Build history of the part. All positions in model axes, mm. A direction names the side the tool comes from. Round coordinates to 2 decimals unless told otherwise and drop trailing zeros. Write each loop counter-clockwise with the first axis right and the second up, starting at its lowest first coordinate (ties: lowest second). Pieces come first, ordered by that corner, then holes. Notation, with made-up numbers: (-3.5, -9) -> (19.5, -9) arc R19 cw to (19.5, 19) -> close; hole circle Ø11 at (-21, -36). An arc over 180 degrees is marked (long way). Answer in a Markdown table with one row per item.
```python
from build123d import *

# Parameters (mm, degrees)
F1_DEPTH = 26
F2_DEPTH = 1.6


with BuildPart() as f1:
    # F0 (on Top) → F1 (new body)
    with BuildSketch(Plane.XY):
        with BuildLine():
            ThreePointArc((54.416171, 57.216655), (0, 61.6), (-54.416171, 57.216655))
            ThreePointArc((-54.416171, 57.216655), (-55.980157, 56.335105), (-56.6, 54.650179))
            Line((-56.6, 54.650179), (-56.6, -54.5))
            ThreePointArc((-56.6, -54.5), (-55.838478, -56.338478), (-54, -57.1))
            Line((-54, -57.1), (54, -57.1))
            ThreePointArc((54, -57.1), (55.838478, -56.338478), (56.6, -54.5))
            Line((56.6, -54.5), (56.6, 54.650179))
            ThreePointArc((56.6, 54.650179), (55.980157, 56.335105), (54.416171, 57.216655))
        make_face()
        with BuildLine():
            Line((54, -55.5), (-54, -55.5))
            ThreePointArc((-54, -55.5), (-54.707107, -55.207107), (-55, -54.5))
            Line((-55, -54.5), (-55, 54.650179))
            ThreePointArc((-55, 54.650179), (-54.761599, 55.298228), (-54.160066, 55.637285))
            ThreePointArc((-54.160066, 55.637285), (0, 60), (54.160066, 55.637285))
            ThreePointArc((54.160066, 55.637285), (54.761599, 55.298228), (55, 54.650179))
            Line((55, 54.650179), (55, -54.5))
            ThreePointArc((55, -54.5), (54.707107, -55.207107), (54, -55.5))
        make_face(mode=Mode.SUBTRACT)
    extrude(amount=F1_DEPTH)

    # F0 (on Top) → F2 (join)
    with BuildSketch(Plane.XY):
        with BuildLine():
            ThreePointArc((-55, -54.5), (-54.707107, -55.207107), (-54, -55.5))
            Line((-54, -55.5), (54, -55.5))
            ThreePointArc((54, -55.5), (54.707107, -55.207107), (55, -54.5))
            Line((55, -54.5), (55, 54.650179))
            ThreePointArc((55, 54.650179), (54.761599, 55.298228), (54.160066, 55.637285))
            ThreePointArc((54.160066, 55.637285), (0, 60), (-54.160066, 55.637285))
            ThreePointArc((-54.160066, 55.637285), (-54.761599, 55.298228), (-55, 54.650179))
            Line((-55, 54.650179), (-55, -54.5))
        make_face()
    extrude(amount=F2_DEPTH)


solid = f1.part
```
Q1. Saw through at B-B on y = 49. Write the cut outline in (x, z).
A:
| item | result |
|---|---|
| outline | (-56.6, 0) -> (56.6, 0) -> (56.6, 26) -> (55, 26) -> (55, 1.6) -> (-55, 1.6) -> (-55, 26) -> (-56.6, 26) -> close |
Q2. Two-plate mould, pull along Y, no slides. Class faces 3 (the cylindrical face through (-55.859, -56.318, 12.818)), 4 (the flat face through (56.6, -1, 13)), 5 (the flat face through (1, -55.5, 14)): released by +Y, released by -Y, zero draft, split by the parting line, or undercut.
A:
| item | result |
|---|---|
| face 3 | released by -Y |
| face 4 | zero draft |
| face 5 | undercut |
Q3. Drop flat-ended pins along their axis: P1, Ø3, axis at x = -30, z = 13, coming from the +Y side; P2, Ø3, axis at x = -40, y = 0.5, coming from the +Z side; P3, Ø1, axis at x = 38.5, y = 22.5, coming from the -Z side. Give the stop position or say it passes through.
A:
| item | result |
|---|---|
| P1 | y = 60.4 |
| P2 | z = 1.6 |
| P3 | z = 0 |
Q4. Saw through at C-C on x = -7. Write the cut outline in (y, z).
A:
| item | result |
|---|---|
| outline | (-57.1, 0) -> (61.53, 0) -> (61.53, 26) -> (59.93, 26) -> (59.93, 1.6) -> (-55.5, 1.6) -> (-55.5, 26) -> (-57.1, 26) -> close |
Q5. Wall check: line 1 (X direction, y = -12.5, z = 15.25); line 2 (Y direction, x = 1.5, z = 3.75); line 3 (Z direction, x = 14.5, y = 34). Give the ranges that are in metal, low to high. Write a range as [from, to].
A:
| item | result |
|---|---|
| line 1 | [-56.6, -55], [55, 56.6] |
| line 2 | [-57.1, -55.5], [60, 61.6] |
| line 3 | [0, 1.6] |
Q6. Which spindle directions (+Z, -Z, +X, -X, +Y, -Y) get a long thin tool onto all of the face, cutting with end or side? Do faces 1 (the cylindrical face through (55.997, 56.315, 12.818)), 2 (the flat face through (-55, -1, 14)). Say none if no direction does.
A:
| item | result |
|---|---|
| face 1 | +Z, -Z, +X, +Y |
| face 2 | +Z |
Q7. Saw through at A-A on z = 18. Write the cut outline in (x, y), plus the area to 3 significant figures.
A:
| item | result |
|---|---|
| outline | (-56.6, -54.5) arc R2.6 ccw to (-54, -57.1) -> (54, -57.1) arc R2.6 ccw to (56.6, -54.5) -> (56.6, 54.65) arc R2.6 ccw to (54.42, 57.22) arc R339.96 ccw to (-54.42, 57.22) arc R2.6 ccw to (-56.6, 54.65) -> close; hole (-55, -54.5) arc R1 ccw to (-54, -55.5) -> (54, -55.5) arc R1 ccw to (55, -54.5) -> (55, 54.65) arc R1 ccw to (54.16, 55.64) arc R338.36 ccw to (-54.16, 55.64) arc R1 ccw to (-55, 54.65) -> close |
| area | 714 mm² |
